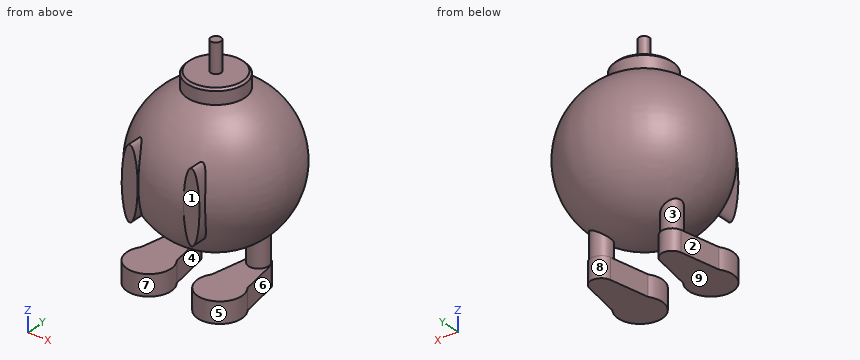
```python
from build123d import *

# Parameters (mm, degrees)
F2_R      = 17.600721
F3_DEPTH  = 50.8
F4_SIZE   = 1.27
F5_R      = 3.193313
F6_DEPTH  = 68.58
F7_R      = 5.852197
F7_R_2    = 6.158231
F8_DEPTH  = 64.77
F10_DEPTH = 12.7
F12_DEPTH = 43.18


with BuildPart() as f1:
    # F0 (on Front) → F1 (revolve)
    with BuildSketch(Plane.XZ):
        with BuildLine():
            ThreePointArc((0, -44.31119), (45.162806, 0.420636), (0, 45.152461))
            Line((0, 45.152461), (0, -44.31119))
        make_face()
    revolve(axis=Axis((0, 0, 0.420636), (0, 0, -1)))

    # F2 (on Top) → F3 (join)
    with BuildSketch(Plane.XY):
        Circle(F2_R)
    extrude(amount=F3_DEPTH)

    # F4
    f4_edges = [f1.edges().sort_by_distance(p)[0] for p in [
        (-17.600721, 0, 50.8),
    ]]
    chamfer(f4_edges, length=F4_SIZE)

    # F5 (on Top) → F6 (join)
    with BuildSketch(Plane.XY):
        Circle(F5_R)
    extrude(amount=F6_DEPTH)

    # F7 (on Top) → F8 (join)
    with BuildSketch(Plane.XY):
        with Locations((-21.764746, 5.852197)):
            Circle(F7_R)
        with Locations((21.764745, 5.852197)):
            Circle(F7_R_2)
    extrude(amount=-F8_DEPTH)

    # F9 (on face) → F10 (join)
    with BuildSketch(Plane(origin=(0, 0, -64.77), x_dir=(1, 0, 0), z_dir=(0, 0, -1))):
        with BuildLine():
            Line((28.323952, -7.020816), (32.743111, 17.168252))
            ThreePointArc((32.743111, 17.168252), (22.03929, 38.695609), (10.879911, 17.40084))
            Line((10.879911, 17.40084), (15.299067, -7.020816))
            ThreePointArc((15.299067, -7.020816), (21.81151, -12.451274), (28.323952, -7.020816))
        make_face()
        with BuildLine():
            Line((-15.286124, -7.020816), (-10.866965, 17.168252))
            ThreePointArc((-10.866965, 17.168252), (-21.570787, 38.695609), (-32.730165, 17.40084))
            Line((-32.730165, 17.40084), (-28.31101, -7.020816))
            ThreePointArc((-28.31101, -7.020816), (-21.798567, -12.451274), (-15.286124, -7.020816))
        make_face()
    extrude(amount=-F10_DEPTH)

    # F11 (on Front) → F12 (join)
    with BuildSketch(Plane.XZ):
        with BuildLine():
            add(Edge.make_bspline(
                [(-19.802049, -21.876966), (-11.238602, -21.876966), (-15.520325, 11.011583), (-19.802049, 43.900133), (-24.083772, 11.011583), (-28.365496, -21.876966), (-19.802049, -21.876966)],
                knots=[0, 0, 0, 2.094395, 2.094395, 4.18879, 4.18879, 6.283185, 6.283185, 6.283185], degree=2, weights=[1, 0.5, 1, 0.5, 1, 0.5, 1]))
        make_face()
        with BuildLine():
            add(Edge.make_bspline(
                [(18.328091, -21.821958), (26.891538, -21.821958), (22.609815, 11.066592), (18.328091, 43.955141), (14.046368, 11.066592), (9.764645, -21.821958), (18.328091, -21.821958)],
                knots=[0, 0, 0, 2.094395, 2.094395, 4.18879, 4.18879, 6.283185, 6.283185, 6.283185], degree=2, weights=[1, 0.5, 1, 0.5, 1, 0.5, 1]))
        make_face()
    extrude(amount=F12_DEPTH)


solid = f1.part
```
The listing builds one solid part. Answer for the finished solid, in the listing's coordinates (mm). Face numbers are marked on the shaded views. A direction names the side the tool comes from. Give positions to 0.01 mm unless a question says otherwise; leave off trailing zeros. Write each loop counter-clockwise with the first axis right and the second up, starting at its lowest first coordinate (ties: lowest second). Pieces come first, ordered by that corner, then holes. Notation, with made-up numbers: (66, 14.5) - (117, 14.5) arc R28 ccw to (117, 32.5) - close; hole circle Ø6 at (-35, 9). An arc over 180 degrees is marked (long way). Use one line per item in the form item = value. Start each with the question number.
1) A tool of negligible diameter and unlimited length cuts with its end or side. For the marked faces 1, 2, 3, 4 and 5, from which of +Z, -Z, +X, -X, +Y, -Y can it reach the whole face along a straight path? Write none if from no direction.
2) Find section B-B on z = 43.5. Determine the outline of the cut face in (x, y).
3) Find section A-A on z = -50. Determine the outline of the cut face in (x, y), plus the area to 3 significant figures.
4) Consider line 1 along Z through (x, y) = (25, -20); line 2 along Z through (x, y) = (29, 3); line 3 along X through (y, z) = (34.5, 24). Determine where each line is inside the solid, lowest interval first. Write a range as from..to.
5) The mould has two halves that part along X. Classify the marked faces 6, 7, 8 and 9: pulls with the +X half, pulls with the -X half, needs draft (parallel to the pull), parting line crosses it, or undercut.
6) Flat-ended cylindrical pins translate along their axes: pin 1 Ø8 at (x, y) = (23.5, -21) entering from +Z; pin 2 Ø11 at (x, z) = (-19, 9) entering from -Y; pin 3 Ø1 at (y, z) = (-16.5, -0.5) entering from -X. Find the tip coordinate at first contact, or state that the pin passes through.
7) Find section C-C on y = -31.5. Count the separate pieces of the cut face and the enclosed holes in it, plus the area to 3 significant figures.
Geometry results:
q1.face_1 = +Z, -Z, +X, -Y
q1.face_2 = -Z, -X, +Y
q1.face_3 = none
q1.face_4 = -Z, +Y
q1.face_5 = -Z
q2.outline = circle Ø35.2 at (0, 0)
q3.outline = circle Ø11.7 at (-21.76, 5.85); circle Ø12.32 at (21.76, 5.85)
q3.area = 227 mm2
q4.line_1 = -64.77..-52.07, -31.26..32.1
q4.line_2 = -64.77..-52.07, -33.87..34.71
q4.line_3 = -16.96..16.96
q5.face_6 = pulls with the +X half
q5.face_7 = undercut
q5.face_8 = undercut
q5.face_9 = needs draft
q6.pin_1 = 36.02
q6.pin_2 = -43.18
q6.pin_3 = -42.22
q7.separate_pieces = 3
q7.enclosed_holes = 0
q7.area = 3,880 mm2
